```python
from build123d import *

# Parameters (mm, degrees)
SKETCH1_W                    = 90.805
SKETCH1_H                    = 44.45
BASE_FLANGE1_DEPTH           = 3.175
EDGE_FLANGE1_STRIP_W         = 14.7
EDGE_FLANGE1_STRIP_H         = 3.175
EDGE_FLANGE1_STRIP_CUT_DEPTH = 44.45
EDGE_FLANGE1_DEPTH           = 44.45
CUT_EXTRUDE1_DEPTH           = 107.396140203
CUT_EXTRUDE1_DEPTH_BACK      = 3.175
M6_CLEARANCE_HOLE3_D         = 7


# Sheet-metal steps are written as plain solids
with BuildPart() as part:
    # Sketch1 → Base-Flange1 (new body)
    with BuildSketch(Plane.XY):
        Rectangle(SKETCH1_W, SKETCH1_H)
    extrude(amount=BASE_FLANGE1_DEPTH)

    # Edge-Flange1 strip (across the edge) → Edge-Flange1 strip cut (cut)
    with BuildSketch(Plane(origin=(-45.4025, 22.225, 3.175), x_dir=(1, 0, 0), z_dir=(0, -1, 0))):
        with Locations((-3.175, -1.5875)):
            Rectangle(EDGE_FLANGE1_STRIP_W, EDGE_FLANGE1_STRIP_H)
    extrude(amount=EDGE_FLANGE1_STRIP_CUT_DEPTH, mode=Mode.SUBTRACT)

    # Edge-Flange1 section (across the edge) → Edge-Flange1 (add)
    with BuildSketch(Plane(origin=(-45.4025, 22.225, 3.175), x_dir=(1, 0, 0), z_dir=(0, -1, 0))):
        with BuildLine():
            Line((0, 1), (0, 47.625))
            Line((0, 47.625), (3.175, 47.625))
            Line((3.175, 47.625), (3.175, 1))
            ThreePointArc((3.175, 1), (3.467893219, 0.292893219), (4.175, 0))
            Line((4.175, 0), (4.175, -3.175))
            ThreePointArc((4.175, -3.175), (1.222829189, -1.952170811), (0, 1))
        make_face()
    extrude(amount=EDGE_FLANGE1_DEPTH)

    # Sketch9 → Cut-Extrude1 (cut, two sides: drawn at the far end of the back side and taken through both)
    with BuildSketch(Plane.ZY.offset(45.4025).offset(-CUT_EXTRUDE1_DEPTH_BACK)):
        Polygon((50.8, 167.227851822), (50.8, 22.225), (50.8, 18.96237), (4.175, -22.225), (-104.498494033, -118.224472556), (150.247183568, -256.81721367), (305.545677601, 28.635110708), align=None)
    extrude(amount=CUT_EXTRUDE1_DEPTH + CUT_EXTRUDE1_DEPTH_BACK, mode=Mode.SUBTRACT)

    # M6 Clearance Hole3 (through all)
    with Locations(Plane.XY.offset(3.175)):
        with Locations((1.5875, 0)):
            Hole(M6_CLEARANCE_HOLE3_D / 2)


solid = part.part
```
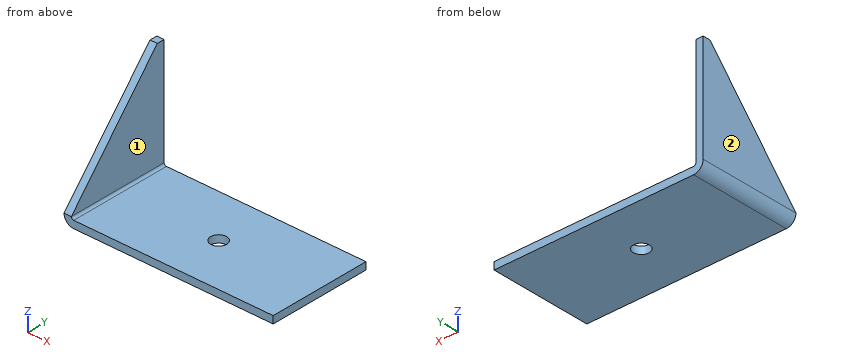
For this review, take the finished solid that the model builds, in its own axes (mm). Face numbers are marked on the shaded views. A direction names the side the tool comes from. Round coordinates to 2 decimals unless told otherwise and drop trailing zeros. Write each loop counter-clockwise with the first axis right and the second up, starting at its lowest first coordinate (ties: lowest second). Pieces come first, ordered by that corner, then holes. Notation, with made-up numbers: (-14, 15.25) - (24, 15.25) arc R30 cw to (24, 39.25) - close; hole circle Ø2 at (72.5, -16). An arc over 180 degrees is marked (long way). Write each question's results on one line, items separated by ' | '.
Item 1: To check wall thickness, follow line 1 along Z through (x, y) = (37.5, -20) (3 decimals); line 2 along X through (y, z) = (5, 30.5). State the ranges of each line that lie inside material, in increasing order. Write a range as from..to.
Calculated:
line 1: z = 0..3.175 | line 2: x = -45.4..-42.23
Item 2: For pin 1 (13.5 mm diameter, centred on y = -9.5, z = 28, fed in from +X); pin 2 (12 mm diameter, centred on x = 29.5, y = 17.5, fed in from +Z) (3 decimals), all flat-tipped, find the tip position at first contact; note any pin that passes through.
Calculated:
pin 1: stops at x = -42.23 | pin 2: stops at z = 3.175
Item 3: For the marked faces 1 and 2, list the 3-axis set-ups (+Z, -Z, +X, -X, +Y, -Y) from which the entire face can be reached by the end or side of a thin tool; tool diameter is ignored.
Calculated:
face 1: +Z, +X, +Y, -Y | face 2: +Z, -Z, -X, +Y, -Y
Item 4: Take a section at C-C on z = 32. State the section outline as (x, y) points (1 decimal).
Calculated:
outline: (-45.4, 2.4) - (-42.2, 2.4) - (-42.2, 22.2) - (-45.4, 22.2) - close
Item 5: Take a section at B-B on x = -34. State the section outline as (y, z) points (3 decimals).
Calculated:
outline: (-22.225, 0) - (22.225, 0) - (22.225, 3.175) - (-22.225, 3.175) - close
